Geometry check sheet. Reference: the model listing, model coordinates, mm. A direction names the side the tool comes from. Coordinates: 2 decimals unless noted, no trailing zeros. Loops run counter-clockwise (first coordinate to the right, second up) from the corner with the lowest first, then second, coordinate; pieces in that order, holes last. Notation, with made-up numbers: M 89,75 L 110,75 A23 ccw 110,87 Z; hole C 62.5,-16 d6. An arc over 180 degrees is marked long. One line per question, with ' | ' between items. Start each with the question number.
from build123d import *

# Parameters (mm, degrees)
F0_W     = 21.1988506515
F0_H     = 22
F0_R     = 8.7104848274
F1_DEPTH = 11
F2_DEPTH = 25
F3_W     = 2
F3_H     = 22
F4_DEPTH = 4
F6_DEPTH = 22.001
F7_R     = 2
F8_DEPTH = 1


with BuildPart() as f1:
    # F0 (on Top) → F1 (new body)
    with BuildSketch(Plane.XY):
        with Locations((0, -0.4590692324)):
            Rectangle(F0_W, F0_H)
        with Locations((0, -0.4590692324)):
            Circle(F0_R, mode=Mode.SUBTRACT)
    extrude(amount=-F1_DEPTH)

    # F2 (add): a face of the model
    f2_faces = [f1.faces().sort_by_distance(p)[0] for p in [
        (10.5994253258, -0.4590692324, -5.5),
    ]]
    extrude(f2_faces, amount=F2_DEPTH)

    # F3 (on face) → F4 (cut)
    with BuildSketch(Plane.XY):
        with Locations((32.5994253258, -0.4590692324)):
            Rectangle(F3_W, F3_H)
        with BuildLine():
            Line((-1.8565698992, -11.4590692324), (2.0946341101, -11.4590692324))
            Line((2.0946341101, -11.4590692324), (2.0946341101, -8.9139526659))
            ThreePointArc((2.0946341101, -8.9139526659), (0.1222177802, -9.168696592), (-1.8565698992, -8.9693979063))
            Line((-1.8565698992, -8.9693979063), (-1.8565698992, -11.4590692324))
        make_face()
        with BuildLine():
            Line((2.0946341101, 7.995814201), (2.0946341101, 10.5409307676))
            Line((2.0946341101, 10.5409307676), (-1.8565698992, 10.5409307676))
            Line((-1.8565698992, 10.5409307676), (-1.8565698992, 8.0512594415))
            ThreePointArc((-1.8565698992, 8.0512594415), (0.1222177802, 8.2505581271), (2.0946341101, 7.995814201))
        make_face()
    extrude(amount=-F4_DEPTH, mode=Mode.SUBTRACT)

    # F5 (on face) → F6 (cut, through all)
    with BuildSketch(Plane.XZ.offset(11.4590692324)):
        Polygon((19.8470297179, 0), (16.8470297179, 0), (13.192070817, -6.330574516), (23.5019886189, -6.330574516), align=None)
    extrude(amount=-F6_DEPTH, mode=Mode.SUBTRACT)

    # F7 (on face) → F8 (join)
    with BuildSketch(Plane.YZ.offset(35.5994253258)):
        with Locations((-2.064286964, -5.0933435559)):
            Circle(F7_R)
    extrude(amount=F8_DEPTH)


solid = f1.part
1. Depth check by flat-ended pin: pin 1 Ø1.3 at (x, y) = (-0.5, -10) entering from +Z; pin 2 Ø8 at (x, y) = (0.5, -5) entering from -Z; pin 3 Ø1.2 at (y, z) = (8.5, -1.5) entering from +X. Enter the tip coordinate at first touch or a pass-through.
2. Sectioned sample at C-C (y = 8.75). Record the cut outline in (x, z).
3. Thickness scan on line 1 (Y direction, x = 0, z = -5.75); line 2 (X direction, y = -8.5, z = -0.5); line 3 (X direction, y = -7.25, z = -4.25). Record the ranges inside material, lowest first.
4. Draft check along Z on faces 3 (the flat face through (-1.857, 9, -2)), 4 (the flat face through (0, 9, -4)), 5 (the flat face through (18, -1, -6.331)), 6 (the flat face through (21.7, -0.61, -3.21)). Enter one of: +Z half, -Z half, draft (parallel to the pull), parting line (faces both ways), or undercut.
5. Sectioned sample at B-B (x = 0). Record the cut outline in (y, z).
6. Tool access check on faces 1 (the flat face through (26, -1, 0)), 2 (the flat face through (31.599, -1, -2)). Record the directions out of +Z, -Z, +X, -X, +Y, -Y that give a thin tool (end or side, any length) a straight path to the whole face; none if there is none.
7. Sectioned sample at D-D (y = 0.5). Record the cut outline in (x, z), and give its area (3 significant figures).
8. Sectioned sample at A-A (z = -5.75). Record the cut outline in (x, y), and give its area (3 significant figures).
Result:
1) pin 1: stops at z = -4 | pin 2: passes through | pin 3: stops at x = 35.6
2) outline: M -10.6,-11 L 35.6,-11 L 35.6,0 L 33.6,0 L 33.6,-4 L 31.6,-4 L 31.6,0 L 19.85,0 L 23.5,-6.33 L 13.19,-6.33 L 16.85,0 L 2.09,0 L 2.09,-4 L -1.86,-4 L -1.86,0 L -10.6,0 Z
3) line 1: y = -11.46 to -9.17, 8.25 to 10.54 | line 2: x = -10.6 to -3.35, 3.35 to 16.56, 20.14 to 31.6, 33.6 to 35.6 | line 3: x = -10.6 to -5.45, 5.45 to 14.39, 22.3 to 35.6
4) face 3: draft | face 4: +Z half | face 5: undercut | face 6: undercut
5) outline: M -11.46,-11 L -9.17,-11 L -9.17,-4 L -11.46,-4 Z; M 8.25,-11 L 10.54,-11 L 10.54,-4 L 8.25,-4 Z
6) face 1: +Z, +X, -X, +Y, -Y | face 2: +Z, +Y, -Y
7) outline: M -10.6,-11 L -8.66,-11 L -8.66,0 L -10.6,0 Z; M 8.66,-11 L 35.6,-11 L 35.6,0 L 33.6,0 L 33.6,-4 L 31.6,-4 L 31.6,0 L 19.85,0 L 23.5,-6.33 L 13.19,-6.33 L 16.85,0 L 8.66,0 Z | area: 268 mm2
8) outline: M -10.6,-11.46 L 13.53,-11.46 L 13.53,10.54 L -10.6,10.54 Z; M 23.17,-11.46 L 35.6,-11.46 L 35.6,-3.95 L 36.6,-3.95 L 36.6,-0.18 L 35.6,-0.18 L 35.6,10.54 L 23.17,10.54 Z; hole C 0,-0.46 d17.42 | area: 570 mm2
